Can you work these out from the model? Positions are in its coordinate system, mm. A direction names the side the tool comes from. Round coordinates to 2 decimals unless told otherwise and drop trailing zeros. Order: outer loops, then holes, each group sorted by start corner. A loop starts at its lowest first (then second) coordinate and runs counter-clockwise, first axis right, second up.
from build123d import *

# Parameters (mm, degrees)
SKETCH1_W               = 95.2
SKETCH1_H               = 205.7
BOSS_EXTRUDE1_DEPTH     = 240
SKETCH2_W               = 228.6
SKETCH2_H               = 83.8
CUT_EXTRUDE1_DEPTH      = 194.3
FILLET1_R               = 1
SKETCH3_R               = 18.5
CUT_EXTRUDE2_DEPTH      = 331.114419558
SKETCH4_W               = 47
SKETCH4_H               = 47
BOSS_EXTRUDE2_DEPTH     = 6.3
SKETCH6_W               = 47
SKETCH6_H               = 47
BOSS_EXTRUDE3_DEPTH     = 6.3
CUT_EXTRUDE3_DEPTH      = 332.986053924
CUT_EXTRUDE3_DEPTH_BACK = 332.986053924
SKETCH7_R               = 18.5
CUT_EXTRUDE4_DEPTH      = 332.986053924
CUT_EXTRUDE4_DEPTH_BACK = 332.986053924
SKETCH8_R               = 23.5
CUT_EXTRUDE5_DEPTH      = 332.986053924
CUT_EXTRUDE5_DEPTH_BACK = 332.986053924
SKETCH9_R               = 12
SKETCH10_W              = 30
SKETCH10_H              = 30
BOSS_EXTRUDE5_DEPTH     = 2.3
SKETCH11_W              = 30
SKETCH11_H              = 30
BOSS_EXTRUDE6_DEPTH     = 2.3
CUT_EXTRUDE6_DEPTH      = 332.986053924
CUT_EXTRUDE6_DEPTH_BACK = 332.986053924
SKETCH12_R              = 12
CUT_EXTRUDE7_DEPTH      = 332.986053924
CUT_EXTRUDE7_DEPTH_BACK = 332.986053924
SKETCH14_R              = 4
SKETCH15_W              = 34
SKETCH15_H              = 10
BOSS_EXTRUDE7_DEPTH     = 2
SKETCH17_W              = 34
SKETCH17_H              = 10
BOSS_EXTRUDE14_DEPTH    = 2
SKETCH18_W              = 24
SKETCH18_H              = 6
BOSS_EXTRUDE17_DEPTH    = 2
SKETCH19_W              = 24
SKETCH19_H              = 6
BOSS_EXTRUDE18_DEPTH    = 2
SKETCH20_W              = 15
SKETCH20_H              = 160
BOSS_EXTRUDE19_DEPTH    = 200
SKETCH21_R              = 6
CUT_EXTRUDE8_DEPTH      = 20
BOSS_EXTRUDE20_DEPTH    = 70


with BuildPart() as part:
    # Sketch1 → Boss-Extrude1 (new body)
    with BuildSketch(Plane(origin=(0, 0, 0), x_dir=(0, 0, -1), z_dir=(1, 0, 0))):
        with Locations((47.6, 102.85)):
            Rectangle(SKETCH1_W, SKETCH1_H)
    extrude(amount=-BOSS_EXTRUDE1_DEPTH)

    # Sketch2 → Cut-Extrude1 (cut)
    with BuildSketch(Plane.XZ):
        with Locations((-120, -47.6)):
            Rectangle(SKETCH2_W, SKETCH2_H)
    extrude(amount=-CUT_EXTRUDE1_DEPTH, mode=Mode.SUBTRACT)

    # Fillet1
    fillet1_edges = [part.edges().sort_by_distance(p)[0] for p in [
        (-240, 102.85, -95.2),
        (-240, 205.7, -47.6),
        (-240, 102.85, 0),
        (0, 205.7, -47.6),
        (0, 102.85, -95.2),
        (0, 102.85, 0),
        (-120, 205.7, 0),
        (-120, 205.7, -95.2),
    ]]
    fillet(fillet1_edges, radius=FILLET1_R)

    # Sketch3 → Cut-Extrude2 (cut, through all)
    with BuildSketch(Plane.XY):
        with Locations((-120, 107)):
            Circle(SKETCH3_R)
    extrude(amount=-CUT_EXTRUDE2_DEPTH, mode=Mode.SUBTRACT)

    # Sketch4 → Boss-Extrude2 (add)
    with BuildSketch(Plane.XY):
        with Locations((-120, 107)):
            Rectangle(SKETCH4_W, SKETCH4_H)
    extrude(amount=BOSS_EXTRUDE2_DEPTH)

    # Sketch6 → Boss-Extrude3 (add)
    with BuildSketch(Plane(origin=(0, 0, -95.2), x_dir=(-1, 0, 0), z_dir=(0, 0, -1))):
        with Locations((120, 107)):
            Rectangle(SKETCH6_W, SKETCH6_H)
    extrude(amount=BOSS_EXTRUDE3_DEPTH)

    # Sketch7 → Cut-Extrude3 (cut, two sides: drawn at the far end of the back side and taken through both)
    with BuildSketch(Plane.XY.offset(-CUT_EXTRUDE3_DEPTH_BACK)):
        with Locations((-120, 107)):
            Circle(SKETCH7_R)
    extrude(amount=CUT_EXTRUDE3_DEPTH + CUT_EXTRUDE3_DEPTH_BACK, mode=Mode.SUBTRACT)

    # Sketch8 → Cut-Extrude4 (cut, two sides: drawn at the far end of the back side and taken through both)
    with BuildSketch(Plane.XY.offset(-CUT_EXTRUDE4_DEPTH_BACK)):
        with Locations((-120, -18.2)):
            Circle(SKETCH8_R)
    extrude(amount=CUT_EXTRUDE4_DEPTH + CUT_EXTRUDE4_DEPTH_BACK, mode=Mode.SUBTRACT)

    # Sketch9 → Cut-Extrude5 (cut, two sides: drawn at the far end of the back side and taken through both)
    with BuildSketch(Plane.XY.offset(-CUT_EXTRUDE5_DEPTH_BACK)):
        with Locations((-120, 162)):
            Circle(SKETCH9_R)
    extrude(amount=CUT_EXTRUDE5_DEPTH + CUT_EXTRUDE5_DEPTH_BACK, mode=Mode.SUBTRACT)

    # Sketch10 → Boss-Extrude5 (add)
    with BuildSketch(Plane.XY):
        with Locations((-120, 162)):
            Rectangle(SKETCH10_W, SKETCH10_H)
    extrude(amount=BOSS_EXTRUDE5_DEPTH)

    # Sketch11 → Boss-Extrude6 (add)
    with BuildSketch(Plane(origin=(0, 0, -95.2), x_dir=(-1, 0, 0), z_dir=(0, 0, -1))):
        with Locations((120, 162)):
            Rectangle(SKETCH11_W, SKETCH11_H)
    extrude(amount=BOSS_EXTRUDE6_DEPTH)

    # Sketch12 → Cut-Extrude6 (cut, two sides: drawn at the far end of the back side and taken through both)
    with BuildSketch(Plane.XY.offset(-CUT_EXTRUDE6_DEPTH_BACK)):
        with Locations((-120, 162)):
            Circle(SKETCH12_R)
    extrude(amount=CUT_EXTRUDE6_DEPTH + CUT_EXTRUDE6_DEPTH_BACK, mode=Mode.SUBTRACT)

    # Sketch14 → Cut-Extrude7 (cut, two sides: drawn at the far end of the back side and taken through both)
    with BuildSketch(Plane.XY.offset(-CUT_EXTRUDE7_DEPTH_BACK)):
        with Locations((-30, 7)):
            Circle(SKETCH14_R)
        with Locations((-210, 7)):
            Circle(SKETCH14_R)
    extrude(amount=CUT_EXTRUDE7_DEPTH + CUT_EXTRUDE7_DEPTH_BACK, mode=Mode.SUBTRACT)

    # Sketch15 → Boss-Extrude7 (add)
    with BuildSketch(Plane(origin=(0, 0, -101.5), x_dir=(-1, 0, 0), z_dir=(0, 0, -1))):
        with Locations((120, 93.35)):
            Rectangle(SKETCH15_W, SKETCH15_H)
        with Locations((120, 120.65)):
            Rectangle(SKETCH15_W, SKETCH15_H)
    extrude(amount=BOSS_EXTRUDE7_DEPTH)

    # Sketch17 → Boss-Extrude14 (add)
    with BuildSketch(Plane.XY.offset(6.3)):
        with Locations((-120, 93.35)):
            Rectangle(SKETCH17_W, SKETCH17_H)
        with Locations((-120, 120.65)):
            Rectangle(SKETCH17_W, SKETCH17_H)
    extrude(amount=BOSS_EXTRUDE14_DEPTH)

    # Sketch18 → Boss-Extrude17 (add)
    with BuildSketch(Plane.XY.offset(2.3)):
        with Locations((-120, 152.5)):
            Rectangle(SKETCH18_W, SKETCH18_H)
        with Locations((-120, 171.5)):
            Rectangle(SKETCH18_W, SKETCH18_H)
    extrude(amount=BOSS_EXTRUDE17_DEPTH)

    # Sketch19 → Boss-Extrude18 (add)
    with BuildSketch(Plane(origin=(0, 0, -97.5), x_dir=(-1, 0, 0), z_dir=(0, 0, -1))):
        with Locations((120, 152.5)):
            Rectangle(SKETCH19_W, SKETCH19_H)
        with Locations((120, 171.5)):
            Rectangle(SKETCH19_W, SKETCH19_H)
    extrude(amount=BOSS_EXTRUDE18_DEPTH)

    # Sketch20 → Boss-Extrude19 (add)
    with BuildSketch(Plane(origin=(0, 0, -95.2), x_dir=(-1, 0, 0), z_dir=(0, 0, -1))):
        with Locations((190.5, 155)):
            Rectangle(SKETCH20_W, SKETCH20_H)
    extrude(amount=BOSS_EXTRUDE19_DEPTH)

    # Sketch21 → Cut-Extrude8 (cut)
    with BuildSketch(Plane.ZY.offset(198)):
        with Locations(Location((-277.7, 211.5, 0), (0, 0, 270))):
            Circle(SKETCH21_R)
        with Locations(Location((-197.7, 211.5, 0), (0, 0, 270))):
            Circle(SKETCH21_R)
        with Locations(Location((-277.7, 111.5, 0), (0, 0, 270))):
            Circle(SKETCH21_R)
        with Locations(Location((-197.7, 111.5, 0), (0, 0, 270))):
            Circle(SKETCH21_R)
    extrude(amount=-CUT_EXTRUDE8_DEPTH, mode=Mode.SUBTRACT)

    # Sketch22 → Boss-Extrude20 (add)
    with BuildSketch(Plane(origin=(0, 205.7, 0), x_dir=(1, 0, 0), z_dir=(0, 1, 0))):
        Polygon((-183, 295.2), (-225, 94.2), (-213.762423012, 94.2), (-183, 241.420167273), align=None)
    extrude(amount=-BOSS_EXTRUDE20_DEPTH)


solid = part.part
(1) I want a section at D-D, the plane z = -111. List the corners of the cut face in (x, y) for me, plus the area to 3 significant figures.
(2) On a 3-axis mill with a long thin cutter (end or side, diameter ignored), from which of +Z, -Z, +X, -X, +Y, -Y can I reach the whole of each face in a straight line? I mean faces 1 (the face through (-120, 93, -103.5)), 2 (the face through (-120, 120, 6.3)), 3 (the face through (-190, 75, -194)), 4 (the face through (-122, 74, -5.7)). Say none if no direction works.
(3) I want a section at C-C, the plane z = -22. List the corners of the cut face in (x, y) for me, plus the area to 3 significant figures.
(4) If we mould it in two halves opening along Z, with no side actions, what happens to faces 5 (the face through (-212.95, 9.7, -2.89)), 6 (the face through (-190.6, 115.92, -193.64)), 7 (the face through (-120, 121, 8.3))? For each: pulls with the +Z half, pulls with the -Z half, needs draft (parallel to the pull), parting line crosses it, or undercut.
(5) I want a section at B-B, the plane x = -30. List the corners of the cut face in (y, z) for me, plus the area to 3 significant figures.
(6) I'm going to push flat-ended pins straight in: pin 1 Ø5 at (x, y) = (-153.5, 32) entering from +Z; pin 2 Ø0.7 at (x, z) = (-118.5, -97) entering from +Y; pin 3 Ø7 at (x, z) = (-123, -97.5) entering from -Y. Where does each tip first touch, or does it pass through?
(7) Please list where these lines run through material, in increasing order: probe 1 along Y at (x, z) = (-194.5, -277.7); probe 2 along X at (y, z) = (7, -2); probe 3 along Y at (x, z) = (-120, -92.5).
(8) I want a section at A-A, the plane y = 19.5. List the corners of the cut face in (x, z) for me.
Ans:
1. outline: (-221.49, 135.7) - (-210.25, 135.7) - (-210.25, 205.7) - (-221.49, 205.7) - close; (-198, 75) - (-183, 75) - (-183, 235) - (-198, 235) - close
1. area: 3,190 mm2
2. face 1: -Z, +X, +Y, -Y
2. face 2: none
2. face 3: -Z, +X, -X, -Y
2. face 4: -Y
3. outline: (-240, 0) - (-234.3, 0) - (-234.3, 194.3) - (-5.7, 194.3) - (-5.7, 0) - (0, 0) - (0, 204.7) arc R1 ccw to (-1, 205.7) - (-239, 205.7) arc R1 ccw to (-240, 204.7) - close
3. area: 4,950 mm2
4. face 5: needs draft
4. face 6: undercut
4. face 7: pulls with the +Z half
5. outline: (0, -95.2) - (3, -95.2) - (3, -89.5) - (0, -89.5) - close; (0, -5.7) - (3, -5.7) - (3, 0) - (0, 0) - close; (11, -95.2) - (204.7, -95.2) arc R1 ccw to (205.7, -94.2) - (205.7, -1) arc R1 ccw to (204.7, 0) - (11, 0) - (11, -5.7) - (194.3, -5.7) - (194.3, -89.5) - (11, -89.5) - close
5. area: 3,210 mm2
6. pin 1: stops at z = 0
6. pin 2: stops at y = 177
6. pin 3: stops at y = 4.61
7. probe 1: y = 75 to 105.5, 117.5 to 205.5, 217.5 to 235
7. probe 2: x = -240 to -214, -206 to -34, -26 to 0
7. probe 3: y = 5.3 to 88.5, 125.5 to 150, 174 to 205.7
8. outline: (-240, -94.2) arc R1 ccw to (-239, -95.2) - (-1, -95.2) arc R1 ccw to (0, -94.2) - (0, -1) arc R1 ccw to (-1, 0) - (-239, 0) arc R1 ccw to (-240, -1) - close; hole (-234.3, -89.5) - (-5.7, -89.5) - (-5.7, -5.7) - (-234.3, -5.7) - close
